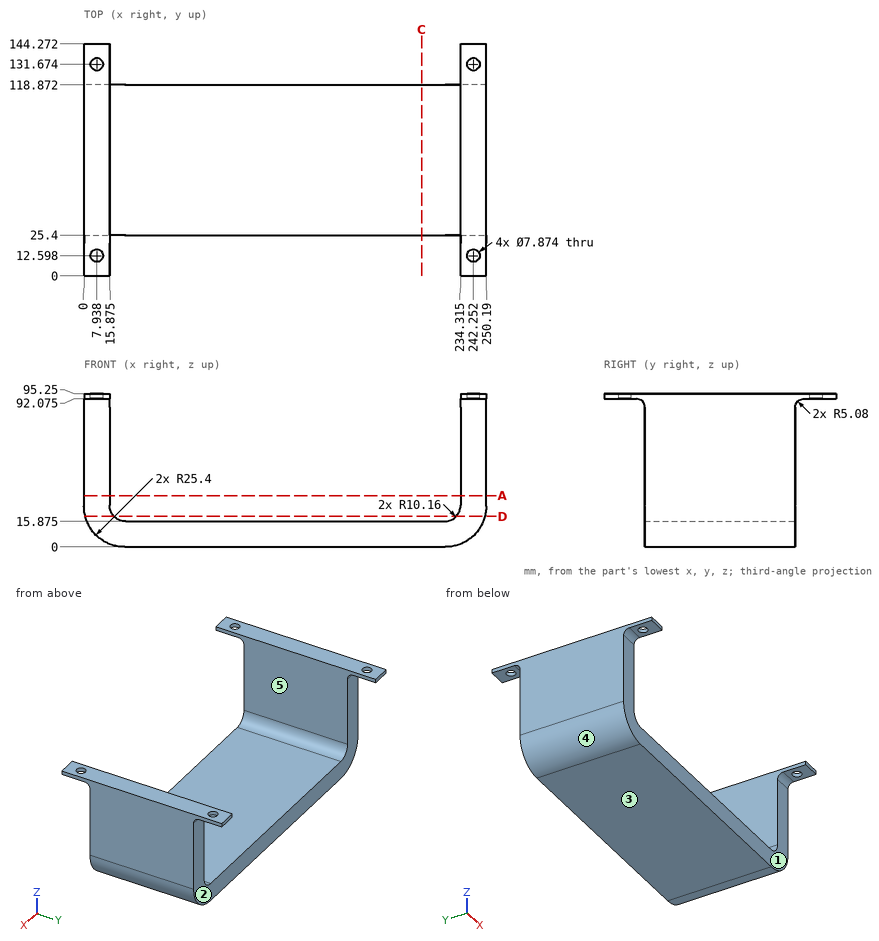
Answer from the drawing. Dimensions are ordinates in mm from the lowest x, y and z of the part. A direction names the side the tool comes from. Round coordinates to 2 decimals unless told otherwise and drop trailing zeros. Write each loop counter-clockwise with the first axis right and the second up, starting at its lowest first coordinate (ties: lowest second). Pieces come first, ordered by that corner, then holes. Notation, with made-up numbers: (-7, 15) - (5, 15) arc R7 ccw to (5, 23) - close; hole circle Ø7 at (7.5, -4.5). An arc over 180 degrees is marked (long way). One line per item, written item: value.
Q1. Find section C-C (x = 210). Determine the outline of the cut face in (y, z) (1 decimal), and give its area (3 significant figures).
The answers:
outline: (25.4, 0) - (118.9, 0) - (118.9, 15.9) - (25.4, 15.9) - close
area: 1,480 mm2
Q2. Straight lines are drawn through the part: line 1 (X direction, y = 67.5, z = 46) (1 decimal); line 2 (Y direction, x = 77, z = 10); line 3 (Z direction, x = 88.5, y = 69) (1 decimal). For each, find the intervals that lie inside material, in ascending order. Write a range as from..to.
The answers:
line 1: x = 0..15.9, 234.3..250.2
line 2: y = 25.4..118.87
line 3: z = 0..15.9
Q3. Which of the six approach directions +Z, -Z, +X, -X, +Y, -Y give full straight-line access (tool end or side, diameter ignored) to the marked faces 1, 2, 3, 4 and 5?
The answers:
face 1: -Z, +X, -X, -Y
face 2: -Z, +X, -X, +Y
face 3: -Z, +X, -X, +Y, -Y
face 4: -Z, -X, +Y, -Y
face 5: +Z, +Y, -Y
Q4. Find section A-A (z = 32). Determine the outline of the cut face in (x, y) (1 decimal), and give its area (3 significant figures).
The answers:
outline: (0, 25.4) - (15.9, 25.4) - (15.9, 118.9) - (0, 118.9) - close; (234.3, 25.4) - (250.2, 25.4) - (250.2, 118.9) - (234.3, 118.9) - close
area: 2,970 mm2
Q5. Find section D-D (z = 19). Determine the outline of the cut face in (x, y) (1 decimal), and give its area (3 significant figures).
The answers:
outline: (0.8, 25.4) - (18.7, 25.4) - (18.7, 118.9) - (0.8, 118.9) - close; (231.5, 25.4) - (249.4, 25.4) - (249.4, 118.9) - (231.5, 118.9) - close
area: 3,340 mm2
Q6. Each of these flat-tipped pins is pushed along its axis until it touches: P1, Ø5, axis at x = 241, y = 7.5, coming from the -Z side (1 decimal); P2, Ø1, axis at x = 190, y = 43.5, coming from the +Z side (1 decimal). Where does it stop, or does it pass through?
The answers:
P1: stops at z = 92.1
P2: stops at z = 15.9
